Verification items for the finished model (mm, model axes). Face numbers are marked on the shaded views. A direction names the side the tool comes from. Give positions to 0.01 mm unless a question says otherwise; leave off trailing zeros. Write each loop counter-clockwise with the first axis right and the second up, starting at its lowest first coordinate (ties: lowest second). Pieces come first, ordered by that corner, then holes. Notation, with made-up numbers: (47, 6.25) -> (79, 6.25) arc R17 ccw to (79, 39.25) -> close; hole circle Ø3 at (-3, 41.5). An arc over 180 degrees is marked (long way). Answer as CSV lines item,"result". Start each with the question number.
1) Tool access check on the marked faces 4 and 5. Record the directions out of +Z, -Z, +X, -X, +Y, -Y that give a thin tool (end or side, any length) a straight path to the whole face; none if there is none.
2) Gauge pin test, flat end, axial feed: pin 1 Ø1.5 at (x, z) = (-1.5, -1.5) entering from -Y. Record the tip position at first contact, or that the pin passes through.
3) Material ranges on L1, parallel to X at y = 0, z = -0.5; L2, parallel to X at y = 2.2, z = 0.9; L3, parallel to Y at x = -10, z = -1.1, recorded low to high.
4) Sectioned sample at D-D on x = -0.5. Record the cut outline in (y, z).
5) Sectioned sample at A-A on z = 0. Record the cut outline in (x, y), and give its area (3 significant figures).
6) Mould release check, pull along X, two halves, no side actions. Record for the marked faces 1, 2 and 3: released by +X, released by -X, zero draft, split by the parting line, or undercut.
7) Sectioned sample at B-B on y = 0. Record the cut outline in (x, z), and give its area (3 significant figures).
8) Sectioned sample at C-C on x = -10. Record the cut outline in (y, z).
```python
from build123d import *

# Parameters (mm, degrees)
SKETCH1_W              = 12
SKETCH1_H              = 2
HEAD_CHAMFER_SIZE      = 1
HEAD_CHAMFER_SIZE2     = 0.577350269
SKETCH21_R             = 0.5
R_CLIP_HOLE_DEPTH      = 4
R_CLIP_HOLE_DEPTH_BACK = 4


with BuildPart() as part:
    # Sketch1 → Body Revolve (revolve)
    with BuildSketch(Plane.XY):
        with Locations((-6, 1)):
            Rectangle(SKETCH1_W, SKETCH1_H)
    revolve(axis=Axis((0, 0, 0), (-1, 0, 0)))

    # Sketch14 → Head Revolve (revolve)
    with BuildSketch(Plane.XY):
        Polygon((0, 0), (1, 0), (1, 2.5), (0.5, 3), (0, 3), align=None)
    revolve(axis=Axis((0, 0, 0), (1, 0, 0)))

    # Head Chamfer
    head_chamfer_edges = [part.edges().sort_by_distance(p)[0] for p in [
        (-12, -2, 0),
    ]]
    head_chamfer_side = [part.faces().sort_by_distance(p)[0] for p in [
        (-6, -2, 0),
    ]]
    chamfer(head_chamfer_edges, length=HEAD_CHAMFER_SIZE, length2=HEAD_CHAMFER_SIZE2, reference=head_chamfer_side[0])

    # Sketch21 → R Clip Hole (cut, two sides)
    with BuildSketch(Plane.XY) as r_clip_hole_sk:
        with Locations((-10, 0)):
            Circle(SKETCH21_R)
    extrude(amount=R_CLIP_HOLE_DEPTH, mode=Mode.SUBTRACT)
    extrude(r_clip_hole_sk.sketch, amount=-R_CLIP_HOLE_DEPTH_BACK, mode=Mode.SUBTRACT)


solid = part.part
```
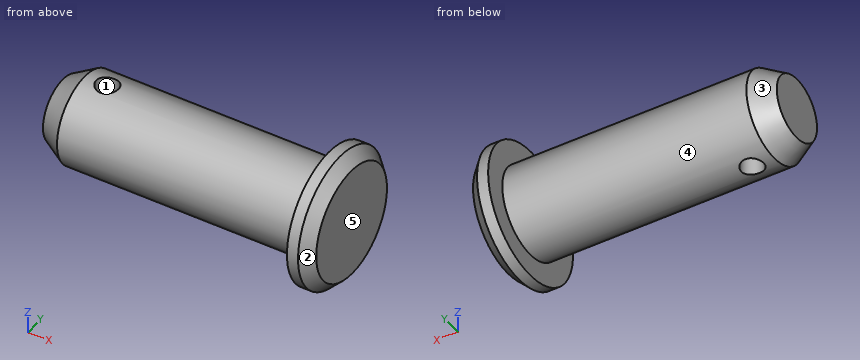
Ans:
1,face 4,"-X"
1,face 5,"+Z, -Z, +X, +Y, -Y"
2,pin 1,"stops at y = -1.85"
3,L1,"x = -12 to -10.5, -9.5 to 1"
3,L2,"x = 0 to 1"
3,L3,"y = -1.67 to -0.5, 0.5 to 1.67"
4,outline,"circle Ø4 at (0, 0)"
5,outline,"(-12, -1.42) -> (-11, -2) -> (0, -2) -> (0, -3) -> (0.5, -3) -> (1, -2.5) -> (1, 2.5) -> (0.5, 3) -> (0, 3) -> (0, 2) -> (-11, 2) -> (-12, 1.42) -> close; hole circle Ø1 at (-10, 0)"
5,area,"52.4 mm²"
6,face 1,"undercut"
6,face 2,"released by +X"
6,face 3,"released by -X"
7,outline,"(-12, -1.42) -> (-11, -2) -> (-10.5, -2) -> (-10.5, 2) -> (-11, 2) -> (-12, 1.42) -> close; (-9.5, -2) -> (0, -2) -> (0, -3) -> (0.5, -3) -> (1, -2.5) -> (1, 2.5) -> (0.5, 3) -> (0, 3) -> (0, 2) -> (-9.5, 2) -> close"
7,area,"49.2 mm²"
8,outline,"(-0.5, -1.94) -> (-0.5, 1.94) arc R2 ccw to start; (0.5, -1.94) arc R2 ccw to (0.5, 1.94) -> close"
